```python
from build123d import *

# Parameters (mm, degrees)
SKETCH1_W               = 101.6
SKETCH1_H               = 50.8
BOSS_EXTRUDE1_DEPTH     = 304.8
CUT_EXTRUDE1_DEPTH      = 314.152231351
CUT_EXTRUDE1_DEPTH_BACK = 314.152231351


with BuildPart() as part:
    # Sketch1 → Boss-Extrude1 (new body)
    with BuildSketch(Plane.XY):
        Rectangle(SKETCH1_W, SKETCH1_H)
    extrude(amount=BOSS_EXTRUDE1_DEPTH)

    # Sketch2 → Cut-Extrude1 (cut, two sides: drawn at the far end of the back side and taken through both)
    with BuildSketch(Plane(origin=(0, 25.4, 0), x_dir=(1, 0, 0), z_dir=(0, 1, 0)).offset(-CUT_EXTRUDE1_DEPTH_BACK)):
        with BuildLine():
            ThreePointArc((25.4, -298.45), (12.7, -285.75), (0, -298.45))
            ThreePointArc((0, -298.45), (0.432742006, -301.737001873), (1.701477372, -304.8))
            Line((1.701477372, -304.8), (23.698522628, -304.8))
            ThreePointArc((23.698522628, -304.8), (24.967257994, -301.737001873), (25.4, -298.45))
        make_face()
        with BuildLine():
            Line((23.698522628, -304.8), (1.701477372, -304.8))
            ThreePointArc((1.701477372, -304.8), (12.7, -311.15), (23.698522628, -304.8))
        make_face()
        with BuildLine():
            Line((25.4, -304.8), (25.4, -298.45))
            ThreePointArc((25.4, -298.45), (24.967257994, -301.737001873), (23.698522628, -304.8))
            Line((23.698522628, -304.8), (25.4, -304.8))
        make_face()
        with BuildLine():
            Line((0, -298.45), (0, -304.8))
            Line((0, -304.8), (1.701477372, -304.8))
            ThreePointArc((1.701477372, -304.8), (0.432742006, -301.737001873), (0, -298.45))
        make_face()
        Polygon((-31.75, -276.0726), (-50.8, -278.749902901), (-50.8, -304.8), (-27.712627225, -304.8), align=None)
    extrude(amount=CUT_EXTRUDE1_DEPTH + CUT_EXTRUDE1_DEPTH_BACK, mode=Mode.SUBTRACT)


solid = part.part
```
Could you check a few things on this model? Use its own coordinates, in mm. A direction names the side the tool comes from. Give positions to 0.01 mm unless a question says otherwise; leave off trailing zeros. Loops run counter-clockwise (first coordinate to the right, second up) from the corner with the lowest first, then second, coordinate; pieces in that order, holes last. Notation, with made-up numbers: (31.25, 9.5) - (72.25, 9.5) arc R35 cw to (72.25, 47.5) - close; hole circle Ø11 at (62.5, -32). An arc over 180 degrees is marked (long way). Use one line per item in the form item = value.
1. I want a section at A-A (y = -20). Please give me the cut outline in (x, z).
Response values:
outline = (-50.8, 0) - (50.8, 0) - (50.8, 304.8) - (25.4, 304.8) - (25.4, 298.45) arc R12.7 cw to (0, 298.45) - (0, 304.8) - (-27.71, 304.8) - (-31.75, 276.07) - (-50.8, 278.75) - close
2. I want a section at B-B (x = 12.7). Please give me the cut outline in (y, z).
Response values:
outline = (-25.4, 0) - (25.4, 0) - (25.4, 285.75) - (-25.4, 285.75) - close
3. I'm going to push flat-ended pins straight in: pin 1 Ø1.9 at (y, z) = (-4.5, 301) entering from -X; pin 2 Ø8 at (x, y) = (-37.5, -9) entering from +Z. Where does each tip first touch, or does it pass through?
Response values:
pin_1 = -28.38
pin_2 = 277.44
4. I need wall thicknesses on probe 1 along Z at (x, y) = (-34, 14); probe 2 along Z at (x, y) = (1.5, 18). Which ranges of each line are inside material? Lowest first, please.
Response values:
probe_1 = 0 to 276.39
probe_2 = 0 to 292.46
5. On a 3-axis mill with a long thin cutter (end or side, diameter ignored), from which of +Z, -Z, +X, -X, +Y, -Y can I reach the whole of each face in a straight line? I mean faces 4 (the face through (38, 0, 304.8)), 5 (the face through (-41.142, -0.356, 277.393)). Say none if no direction works.
Response values:
face_4 = +Z, +X, -X, +Y, -Y
face_5 = +Z, +Y, -Y
6. Thinking about a two-plate mould opening in X: for faces 1 (the face through (50.8, 0, 150)), 2 (the face through (-1, 25.4, 150)), 3 (the face through (0, 0, 302)), which applies, released by +X, released by -X, zero draft, split by the parting line, or undercut?
Response values:
face_1 = released by +X
face_2 = zero draft
face_3 = undercut
